```python
from build123d import *

# Parameters (mm, degrees)
SKETCH1_W           = 180
SKETCH1_H           = 120
BOSS_EXTRUDE1_DEPTH = 100
SKETCH2_W           = 130
SKETCH2_H           = 100
CUT_EXTRUDE1_DEPTH  = 90
CUT_EXTRUDE2_DEPTH  = 17
CUT_EXTRUDE3_DEPTH  = 17
CUT_EXTRUDE4_START  = -100
SKETCH6_W           = 180
SKETCH6_H           = 10
CUT_EXTRUDE4_DEPTH  = 100
SKETCH7_W           = 130
SKETCH7_H           = 10
BOSS_EXTRUDE2_DEPTH = 100


with BuildPart() as part:
    # Sketch1 → Boss-Extrude1 (new body)
    with BuildSketch(Plane(origin=(0, 0, 0), x_dir=(1, 0, 0), z_dir=(0, 1, 0))):
        with Locations((90, 60)):
            Rectangle(SKETCH1_W, SKETCH1_H)
    extrude(amount=BOSS_EXTRUDE1_DEPTH)

    # Sketch2 → Cut-Extrude1 (cut)
    with BuildSketch(Plane(origin=(0, 100, 0), x_dir=(1, 0, 0), z_dir=(0, 1, 0))):
        with Locations((90, 60)):
            Rectangle(SKETCH2_W, SKETCH2_H)
    extrude(amount=-CUT_EXTRUDE1_DEPTH, mode=Mode.SUBTRACT)

    # Sketch3 → Cut-Extrude2 (cut)
    with BuildSketch(Plane(origin=(180, 0, 0), x_dir=(0, 0, -1), z_dir=(1, 0, 0))):
        with BuildLine():
            Line((32, 0), (88, 0))
            ThreePointArc((88, 0), (60, 28), (32, 0))
        make_face()
    extrude(amount=-CUT_EXTRUDE2_DEPTH, mode=Mode.SUBTRACT)

    # Sketch5 → Cut-Extrude3 (cut)
    with BuildSketch(Plane.ZY):
        with BuildLine():
            Line((-88, 0), (-32, 0))
            ThreePointArc((-32, 0), (-60, 28), (-88, 0))
        make_face()
    extrude(amount=-CUT_EXTRUDE3_DEPTH, mode=Mode.SUBTRACT)

    # Sketch6 → Cut-Extrude4 (cut)
    with BuildSketch(Plane(origin=(0, 100, 0), x_dir=(1, 0, 0), z_dir=(0, 1, 0)).offset(CUT_EXTRUDE4_START)):
        with Locations((90, 5)):
            Rectangle(SKETCH6_W, SKETCH6_H)
    extrude(amount=CUT_EXTRUDE4_DEPTH, mode=Mode.SUBTRACT)

    # Sketch7 → Boss-Extrude2 (add)
    with BuildSketch(Plane.XY.offset(-110)):
        with Locations((90, 50)):
            Rectangle(SKETCH7_W, SKETCH7_H)
    extrude(amount=BOSS_EXTRUDE2_DEPTH)


solid = part.part
```
Geometry: final body of the model. Coordinates: model frame, mm. A direction names the side the tool comes from. Round coordinates to 2 decimals unless told otherwise and drop trailing zeros. Loops run counter-clockwise (first coordinate to the right, second up) from the corner with the lowest first, then second, coordinate; pieces in that order, holes last. Notation, with made-up numbers: (47, -4.75) -> (102, -4.75) arc R20 ccw to (102, 25.25) -> close; hole circle Ø1 at (63.25, -13.5). An arc over 180 degrees is marked (long way). Use one line per item in the form item = value.
Item 1: Cut plane B-B on y = 71.5. Output: boundary loops of the cut face in (x, z), then the cut area to 3 significant figures.
Evaluation:
outline = (0, -120) -> (180, -120) -> (180, -10) -> (155, -10) -> (155, -110) -> (25, -110) -> (25, -10) -> (0, -10) -> close
area = 6,800 mm2
Item 2: Access query for faces 1 (the flat face through (163, 11, -60)), 2 (the flat face through (17, 11, -60)), 3 (the flat face through (25, 78, -59)), 4 (the flat face through (89, 10, -61)). Directions: +Z, -Z, +X, -X, +Y, -Y. A direction counts if a zero-diameter tool reaches every point of the face in a straight line with its end or side. Return the directions, or none.
Evaluation:
face_1 = +X, -Y
face_2 = -X, -Y
face_3 = +Z, +Y
face_4 = +Z
Item 3: Contact query for flat-ended pins moving along their axis: pin 1 Ø2 at (x, z) = (53.5, -64.5) entering from +Y; pin 2 Ø17.5 at (x, y) = (77, 25) entering from +Z. Output: stop coordinate, or through.
Evaluation:
pin_1 = 55
pin_2 = -110
Item 4: Cut plane A-A on z = -108. Output: boundary loops of the cut face in (x, y).
Evaluation:
outline = (0, 0) -> (180, 0) -> (180, 100) -> (155, 100) -> (155, 55) -> (25, 55) -> (25, 100) -> (0, 100) -> close; hole (25, 10) -> (155, 10) -> (155, 45) -> (25, 45) -> close
Item 5: Draft query along X for faces 5 (the flat face through (180, 49, -64)), 6 (the flat face through (89, 0, -66)), 7 (the flat face through (89, 55, -61)), 8 (the flat face through (89, 28, -110)). Return one class per face: released by +X, released by -X, zero draft, split by the parting line, or undercut.
Evaluation:
face_5 = released by +X
face_6 = zero draft
face_7 = undercut
face_8 = undercut
Item 6: Cut plane C-C on x = 61. Output: boundary loops of the cut face in (y, z), then the cut area to 3 significant figures.
Evaluation:
outline = (0, -120) -> (100, -120) -> (100, -110) -> (55, -110) -> (55, -10) -> (45, -10) -> (45, -110) -> (10, -110) -> (10, -10) -> (0, -10) -> close
area = 3,000 mm2
Item 7: Material intervals for probe 1 along Y at (x, z) = (133, -82.5); probe 2 along X at (y, z) = (94, -66.5); probe 3 along Z at (x, y) = (56, 14), sorted ascending.
Evaluation:
probe_1 = 0 to 10, 45 to 55
probe_2 = 0 to 25, 155 to 180
probe_3 = -120 to -110
Item 8: Cut plane D-D on z = -60. Output: boundary loops of the cut face in (x, y).
Evaluation:
outline = (0, 28) -> (17, 28) -> (17, 0) -> (163, 0) -> (163, 28) -> (180, 28) -> (180, 100) -> (155, 100) -> (155, 55) -> (25, 55) -> (25, 100) -> (0, 100) -> close; hole (25, 10) -> (155, 10) -> (155, 45) -> (25, 45) -> close
